Design review of the part built by this model. Coordinates are the model's own, in mm. A direction names the side the tool comes from. Coordinates: 2 decimals unless noted, no trailing zeros. Loops run counter-clockwise (first coordinate to the right, second up) from the corner with the lowest first, then second, coordinate; pieces in that order, holes last. Notation, with made-up numbers: (27.5, 52) - (32.5, 52) arc R14 ccw to (32.5, 71) - close; hole circle Ø5 at (-28, 25.25). An arc over 180 degrees is marked (long way). Answer in a Markdown table with one row per item. Add a question column.
(1) We need section A-A, the plane x = 137. Write out the cut boundary in (y, z).
(2) Clearance check with flat-ended pins moving along their axes: pin 1 (8 mm diameter, centred on x = 187.5, z = -12.5, fed in from +Y); pin 2 (1 mm diameter, centred on y = -8.5, z = 29, fed in from +X); pin 3 (1 mm diameter, centred on x = 62, z = 22, fed in from +Y). State where each tip first meets the part, or that it passes through.
(3) To check wall thickness, follow L1, parallel to X at y = 2, z = 0; L2, parallel to Z at x = 137, y = -16; L3, parallel to Z at x = 137, y = 5. State the ranges of each line that lie inside material, in increasing order. Write a range as [from, to].
(4) The part is to be moulded in two halves that separate along Z. For faces 4 (the face through (129.46, 0.41, 3.92)), 5 (the face through (265, 0, 0)), 6 (the face through (130.673, 26.789, 11.107)), say which applies: released by +Z, released by -Z, zero draft, split by the parting line, or undercut.
(5) For faces 1 (the face through (-3, 0, 0)), 2 (the face through (50, -29, 3)), 3 (the face through (0, -8, 8)), list the 3-axis set-ups (+Z, -Z, +X, -X, +Y, -Y) from which the entire face can be reached by the end or side of a thin tool; tool diameter is ignored.
(6) We need section C-C, the plane x = 247. Write out the cut boundary in (y, z).
(7) We need section B-B, the plane x = 110. Write out the cut boundary in (y, z), plus the area to 3 significant figures.
from build123d import *

# Parameters (mm, degrees)
FASE1_SIZE                      = 1
VERRUNDUNG1_R                   = 5
SKIZZE2_R                       = 8.5
SCHNITT_LINEAR_AUSTRAGEN1_DEPTH = 55


with BuildPart() as part:
    # Skizze1 → Rotation1 (revolve)
    with BuildSketch(Plane.XY):
        Polygon((0, 40), (50, 40), (50, 29), (210, 29), (265, 8.981637115), (265, 0), (0, 0), (-3, 0), (-3, 10), (0, 10), align=None)
    revolve(axis=Axis((265, 0, 0), (-1, 0, 0)))

    # Fase1
    fase1_edges = [part.edges().sort_by_distance(p)[0] for p in [
        (50, -40, 0),
    ]]
    chamfer(fase1_edges, length=FASE1_SIZE)

    # Verrundung1
    verrundung1_edges = [part.edges().sort_by_distance(p)[0] for p in [
        (265, -8.981637115, 0),
        (210, -29, 0),
    ]]
    fillet(verrundung1_edges, radius=VERRUNDUNG1_R)

    # Skizze2 → Schnitt-Linear austragen1 (cut, symmetric)
    with BuildSketch(Plane(origin=(0, 0, 0), x_dir=(1, 0, 0), z_dir=(0, 1, 0))):
        with Locations(Location((137, 0, 0), (0, 0, 270))):  # turned: the seam where the file's is
            Circle(SKIZZE2_R)
    extrude(amount=SCHNITT_LINEAR_AUSTRAGEN1_DEPTH, both=True, mode=Mode.SUBTRACT)


solid = part.part
Responses:
| question | item | result |
|---|---|---|
| 1 | outline | (-27.73, -8.5) arc R29 ccw to (27.73, -8.5) - close; (-27.73, 8.5) - (27.73, 8.5) arc R29 ccw to start |
| 2 | pin 1 | stops at y = 27.73 |
| 2 | pin 2 | stops at x = 50 |
| 2 | pin 3 | stops at y = 19.46 |
| 3 | L1 | x = [-3, 128.5], [145.5, 265] |
| 3 | L2 | z = [-24.19, -8.5], [8.5, 24.19] |
| 3 | L3 | z = [-28.57, -8.5], [8.5, 28.57] |
| 4 | face 4 | undercut |
| 4 | face 5 | zero draft |
| 4 | face 6 | split by the parting line |
| 5 | face 1 | +Z, -Z, -X, +Y, -Y |
| 5 | face 2 | +X |
| 5 | face 3 | -X |
| 6 | outline | circle Ø31.07 at (0, 0) |
| 7 | outline | circle Ø58 at (0, 0) |
| 7 | area | 2,640 mm2 |
